from build123d import *

# Parameters (mm, degrees)
FILLET_4_R       = 3
F_4_0MM_4_D      = 4
F_4_0MM_4_DEPTH  = 8
F_4_0MM_4_TIP    = 1.201721238
F_4_0MM_5_D      = 4
F_4_0MM_5_DEPTH  = 7
F_4_0MM_5_TIP    = 1.201721238
F_10_0MM_1_D     = 10
F_10_0MM_1_DEPTH = 1.995696905
F_10_0MM_1_TIP   = 3.004303095


# Read off the part's stored shape, not the designer's step: M16 机械螺纹 螺柱1
with BuildPart() as part:
    # 草图1 → 旋转1 (revolve)
    with BuildSketch(Plane.XY, mode=Mode.PRIVATE) as revolve_1_sk:
        Polygon((0, 0), (0, 8), (27, 8), (27, 8.5), (83, 8.5), (83, 18), (65, 18), (65, 27), (113, 27), (113, 18), (95, 18), (95, 8.5), (180, 8.5), (180, 0), align=None)
    revolve(revolve_1_sk.sketch.rotate(Axis((0, 0, 0), (1, 0, 0)), 90), axis=Axis((0, 0, 0), (1, 0, 0)))

    # 圆角4
    fillet_4_edges = [part.edges().sort_by_distance(p)[0] for p in [
        (95, 0, -8.5),
        (95, 0, -18),
        (83, 0, -18),
        (83, 0, -8.5),
    ]]
    fillet(fillet_4_edges, radius=FILLET_4_R)

    # M16 机械螺纹 螺柱1 outline → M16 机械螺纹 螺柱1 (revolve, cut)
    with BuildSketch(Plane.YX):
        Polygon((8, 1.0825), (6.9175, 0), (8, 0), align=None)
    revolve(axis=Axis((0, 0, 0), (1, 0, 0)), mode=Mode.SUBTRACT)

    # Ø4.0mm 暗销孔4
    with Locations(Plane(origin=(17.1, 8, 0), x_dir=(0, 0, 1), z_dir=(0, 1, 0))):
        with Locations((0, 0)):
            Hole(F_4_0MM_4_D / 2, depth=F_4_0MM_4_DEPTH)
            with Locations((0, 0, -(F_4_0MM_4_DEPTH + F_4_0MM_4_TIP / 2))):  # 118° drill point
                Cone(0, F_4_0MM_4_D / 2, F_4_0MM_4_TIP, mode=Mode.SUBTRACT)

    # Ø4.0mm 暗销孔5
    with Locations(Plane(origin=(180, 0, 0), x_dir=(0, 0, -1), z_dir=(1, 0, 0))):
        with Locations((0, 0)):
            Hole(F_4_0MM_5_D / 2, depth=F_4_0MM_5_DEPTH)
            with Locations((0, 0, -(F_4_0MM_5_DEPTH + F_4_0MM_5_TIP / 2))):  # 118° drill point
                Cone(0, F_4_0MM_5_D / 2, F_4_0MM_5_TIP, mode=Mode.SUBTRACT)

    # Ø10.0mm 暗销孔1
    with Locations(Plane(origin=(164, 8.5, 0), x_dir=(0, 0, 1), z_dir=(0, 1, 0))):
        with Locations((0, 0)):
            Hole(F_10_0MM_1_D / 2, depth=F_10_0MM_1_DEPTH)
            with Locations((0, 0, -(F_10_0MM_1_DEPTH + F_10_0MM_1_TIP / 2))):  # 118° drill point
                Cone(0, F_10_0MM_1_D / 2, F_10_0MM_1_TIP, mode=Mode.SUBTRACT)


solid = part.part
Model file for the job. Use its own axes, mm. A direction names the side the tool comes from. Coordinates: 2 decimals unless noted, no trailing zeros. Write each loop counter-clockwise with the first axis right and the second up, starting at its lowest first coordinate (ties: lowest second). Pieces come first, ordered by that corner, then holes. Notation, with made-up numbers: (47.25, 77) - (70.25, 77) arc R33 ccw to (70.25, 115) - close; hole circle Ø9 at (88, -16.5). An arc over 180 degrees is marked (long way). Write each question's results on one line, items separated by ' | '. Start each with the question number.
1) Cut at A-A (x = 57.5). Write the cut outline in (y, z).
2) 3-axis set-ups, long thin cutter, end or side, ignore diameter. For faces 1 (the face through (159.12, 7.27, 1.08)), 2 (the face through (105.395, -12.165, -13.267)), 3 (the face through (0, 0, 0)), 4 (the face through (14.223, -6.746, 4.301)): which of +Z, -Z, +X, -X, +Y, -Y reach the whole face in a straight line?
3) Cut at B-B (y = -23). Write the cut outline in (x, z), then the cut area to 3 significant figures.
4) Flat gauge pins, fed straight in: P1, Ø5, axis at y = 12.5, z = 15.5, coming from the +X side; P2, Ø2, axis at x = 40.5, y = 2.5, coming from the +Z side; P3, Ø5, axis at x = 67, y = 3, coming from the -Z side. Where does each tip first touch, or does it go through?
5) Mould opens along Y. For faces 5 (the face through (180, 2, 2)), 6 (the face through (164.73, 4.02, 0.47)), 7 (the face through (72.395, -12.165, -13.267)), 8 (the face through (89.34, 26.36, -5.85)) say: pulls with the +Y half, pulls with the -Y half, needs draft (parallel to the pull), parting line crosses it, or undercut.
6) Cut at C-C (y = 21.5). Write the cut outline in (x, z), then the cut area to 3 significant figures.
7) Probe line 1 along Y through (x, z) = (108.5, 0); line 2 along Y through (x, z) = (175.5, 0); line 3 along X through (y, z) = (4, 0). List the from-to ranges inside material, lowest first. Write a range as from..to.
Returned:
1) outline: circle Ø17 at (0, 0)
2) face 1: +Y | face 2: +X | face 3: +Z, -Z, -X, +Y, -Y | face 4: -X
3) outline: (65, -14.14) - (113, -14.14) - (113, 14.14) - (65, 14.14) - close | area: 1,360 mm^2
4) P1: x = 113 | P2: z = 8.37 | P3: z = -27
5) face 5: needs draft | face 6: pulls with the +Y half | face 7: undercut | face 8: parting line crosses it
6) outline: (65, -16.33) - (113, -16.33) - (113, 16.33) - (65, 16.33) - close | area: 1,570 mm^2
7) line 1: -27..-18, -8.5..8.5, 18..27 | line 2: -8.5..-2, 2..8.5 | line 3: 0..15.1, 19.1..163.17, 164.83..180
